Verification items for the finished model (mm, model axes). Give positions to 0.01 mm unless a question says otherwise; leave off trailing zeros. Order: outer loops, then holes, each group sorted by start corner. A loop starts at its lowest first (then second) coordinate and runs counter-clockwise, first axis right, second up.
from build123d import *

# Parameters (mm, degrees)
SKETCH_1_W          = 38
SKETCH_1_H          = 70
SKETCH_1_R          = 1.6
EXTRUDE_1_DEPTH     = 2
FILLET_1_R          = 2
SKETCH_3_W          = 70
SKETCH_3_H          = 38
SKETCH_3_R          = 1.6
EXTRUDE_2_DEPTH     = 2
CUT_EXTRUDE_2_DEPTH = 2
FILLET_3_R          = 2
FILLET_4_R          = 3
CUT_EXTRUDE_3_DEPTH = 2
FILLET_5_R          = 2


with BuildPart() as part:
    # 草图1 → 凸台-拉伸1 (new body)
    with BuildSketch(Plane.XY):
        Rectangle(SKETCH_1_W, SKETCH_1_H)
        with Locations((16, 32)):
            Circle(SKETCH_1_R, mode=Mode.SUBTRACT)
        with Locations((-16, 32)):
            Circle(SKETCH_1_R, mode=Mode.SUBTRACT)
        with Locations((-16, -32)):
            Circle(SKETCH_1_R, mode=Mode.SUBTRACT)
        with Locations((16, -32)):
            Circle(SKETCH_1_R, mode=Mode.SUBTRACT)
    extrude(amount=EXTRUDE_1_DEPTH)

    # 圆角1
    fillet_1_edges = [part.edges().sort_by_distance(p)[0] for p in [
        (19, -35, 1),
        (-19, -35, 1),
        (-19, 35, 1),
        (19, 35, 1),
    ]]
    fillet(fillet_1_edges, radius=FILLET_1_R)

    # 草图3 → 凸台-拉伸2 (add)
    with BuildSketch(Plane.XY.offset(2)):
        Rectangle(SKETCH_3_W, SKETCH_3_H)
        with Locations((32, 16)):
            Circle(SKETCH_3_R, mode=Mode.SUBTRACT)
        with Locations((-32, 16)):
            Circle(SKETCH_3_R, mode=Mode.SUBTRACT)
        with Locations((-32, -16)):
            Circle(SKETCH_3_R, mode=Mode.SUBTRACT)
        with Locations((32, -16)):
            Circle(SKETCH_3_R, mode=Mode.SUBTRACT)
    extrude(amount=-EXTRUDE_2_DEPTH)

    # 草图4 → 切除-拉伸2 (cut)
    with BuildSketch(Plane.XY.offset(2)):
        with BuildLine():
            Line((-10.5, 1.6), (-5.5, 1.6))
            ThreePointArc((-5.5, 1.6), (-3.9, 0), (-5.5, -1.6))
            Line((-5.5, -1.6), (-10.5, -1.6))
            ThreePointArc((-10.5, -1.6), (-12.1, 0), (-10.5, 1.6))
        make_face()
        with BuildLine():
            Line((19.5, 1.6), (24.5, 1.6))
            ThreePointArc((24.5, 1.6), (26.1, 0), (24.5, -1.6))
            Line((24.5, -1.6), (19.5, -1.6))
            ThreePointArc((19.5, -1.6), (17.9, 0), (19.5, 1.6))
        make_face()
    extrude(amount=-CUT_EXTRUDE_2_DEPTH, mode=Mode.SUBTRACT)

    # 圆角3
    fillet_3_edges = [part.edges().sort_by_distance(p)[0] for p in [
        (35, -19, 1),
        (-35, 19, 1),
        (35, 19, 1),
        (-35, -19, 1),
    ]]
    fillet(fillet_3_edges, radius=FILLET_3_R)

    # 圆角4
    fillet_4_edges = [part.edges().sort_by_distance(p)[0] for p in [
        (-19, 19, 1),
        (-19, -19, 1),
        (19, -19, 1),
        (19, 19, 1),
    ]]
    fillet(fillet_4_edges, radius=FILLET_4_R)

    # 草图5 → 切除-拉伸3 (cut)
    with BuildSketch(Plane.XY.offset(2)):
        Polygon((0, 14.222007672), (-11.830337301, 4.6), (11.830337301, 4.6), align=None)
        Polygon((-15, 26.422007672), (-15, 7.177992328), (-3.169662699, 16.8), align=None)
        Polygon((-11.830337301, 29), (0, 19.377992328), (11.830337301, 29), align=None)
        Polygon((15, 26.422007672), (3.169662699, 16.8), (15, 7.177992328), align=None)
    cut_extrude_3 = extrude(amount=-CUT_EXTRUDE_3_DEPTH, mode=Mode.SUBTRACT)

    # 镜向1: 切除-拉伸3 across plane
    add(cut_extrude_3.mirror(Plane.ZX), mode=Mode.SUBTRACT)

    # 圆角5
    fillet_5_edges = [part.edges().sort_by_distance(p)[0] for p in [
        (-11.830337301, 29, 1),
        (11.830337301, 29, 1),
        (0, 19.377992328, 1),
        (-3.169662699, 16.8, 1),
        (-15, 7.177992328, 1),
        (-15, 26.422007672, 1),
        (15, 26.422007672, 1),
        (15, 7.177992328, 1),
        (3.169662699, 16.8, 1),
        (0, 14.222007672, 1),
        (11.830337301, 4.6, 1),
        (-11.830337301, 4.6, 1),
        (11.830337301, -29, 1),
        (-11.830337301, -29, 1),
        (0, -19.377992328, 1),
        (-15, -7.177992328, 1),
        (-3.169662699, -16.8, 1),
        (-15, -26.422007672, 1),
        (15, -7.177992328, 1),
        (15, -26.422007672, 1),
        (3.169662699, -16.8, 1),
        (11.830337301, -4.6, 1),
        (0, -14.222007672, 1),
        (-11.830337301, -4.6, 1),
    ]]
    fillet(fillet_5_edges, radius=FILLET_5_R)


solid = part.part
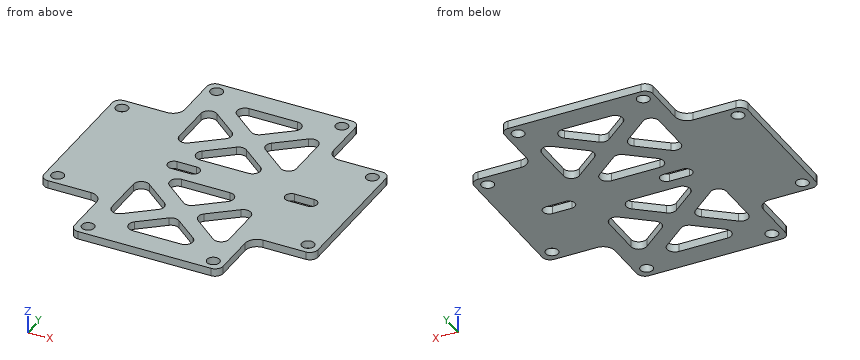
(1) Section check A-A, the plane x = -16. Enter the section's corners in (y, z).
Solved:
outline: (-35, 0) - (-33.6, 0) - (-33.6, 2) - (-35, 2) - close; (-30.4, 0) - (30.4, 0) - (30.4, 2) - (-30.4, 2) - close; (33.6, 0) - (35, 0) - (35, 2) - (33.6, 2) - close
(2) Section check C-C, the plane x = -3. Enter the section's corners in (y, z), then the cut area to 3 significant figures.
Solved:
outline: (-35, 0) - (-29, 0) - (-29, 2) - (-35, 2) - close; (-21.82, 0) - (-11.78, 0) - (-11.78, 2) - (-21.82, 2) - close; (-4.6, 0) - (4.6, 0) - (4.6, 2) - (-4.6, 2) - close; (11.78, 0) - (21.82, 0) - (21.82, 2) - (11.78, 2) - close; (29, 0) - (35, 0) - (35, 2) - (29, 2) - close
area: 82.5 mm2
(3) Section check B-B, the plane y = 0. Enter the section's corners in (x, z), then the cut area to 3 significant figures.
Solved:
outline: (-35, 0) - (-12.1, 0) - (-12.1, 2) - (-35, 2) - close; (-3.9, 0) - (17.9, 0) - (17.9, 2) - (-3.9, 2) - close; (26.1, 0) - (35, 0) - (35, 2) - (26.1, 2) - close
area: 107 mm2
(4) Go/stop test with flat-tipped pins: pin 1 (1 mm diameter, centred on y = -27.5, z = 1, fed in from +X); pin 2 (1 mm diameter, centred on y = 28, z = 1.5, fed in from -X); pin 3 (1 mm diameter, centred on x = -27.5, z = 0.5, fed in from -Y). Record where each tip stops, or that it passes through.
Solved:
pin 1: stops at x = 19
pin 2: stops at x = -19
pin 3: stops at y = -19
(5) Scan lines: line 1 (Y direction, x = -16, z = 1.3); line 2 (X direction, y = 7, z = 1.25); line 3 (Y direction, x = 17, z = 0.3). Record each from-to range of solid material in increasing order.
Solved:
line 1: y = -35 to -33.6, -30.4 to 30.4, 33.6 to 35
line 2: x = -35 to -8.16, 8.16 to 35
line 3: y = -35 to -33.25, -30.75 to 30.75, 33.25 to 35
(6) Section check D-D, the plane z = 0.65. Give the number of separate pieces and of enclosed holes in the cut face, then the cut area to 3 significant figures.
Solved:
separate pieces: 1
enclosed holes: 18
area: 2,940 mm2
